Input: dimensioned drawing with shaded views. Units: mm. Origin: part minimum x, y, z. A direction names the side the tool comes from. Give positions to 0.01 mm unless a question says otherwise; leave off trailing zeros. Order: outer loops, then holes, each group sorted by start corner. A loop starts at its lowest first (then second) coordinate and runs counter-clockwise, first axis right, second up. Notation, with made-up numbers: (52, -1) -> (104, -1) arc R30 cw to (104, 38) -> close; hole circle Ø7 at (69, 21). An arc over 180 degrees is marked (long way). One line per question, with ' | ' between items. Start each with the question number.
(1) Set-up query: the marked faces 5 and 6. Return all of +Z, -Z, +X, -X, +Y, -Y with unobstructed straight access to the full face (end or side cutting, diameter ignored); none if empty.
(2) Mould query, pull axis X, two halves, no side actions, for the marked faces 1, 2, 3 and 4. Classes: +X half, -X half, draft (parallel to the pull), parting line (faces both ways), or undercut.
(3) Section B-B (x = 4.75). Return loops of the section in (y, z), then the cut area to 3 significant figures.
(4) Ray query, L1, parallel to X at y = 0.4, z = 23; L2, parallel to Y at x = 10, z = 41; L3, parallel to Z at x = 12.75, y = 2.9. Return the intervals inside material, ascending.
(5) First-contact query: pin 1 Ø2 at (x, y) = (9, 1.5) entering from -Z; pin 2 Ø3 at (x, z) = (10.5, 23.5) entering from -Y; pin 3 Ø3.5 at (x, y) = (12, 2) entering from +Z. Flat tips, straight axial feed; report the tip coordinate or a pass-through.
(6) Section C-C (y = 2.45). Return loops of the section in (x, z).
(7) Section A-A (z = 40). Return loops of the section in (x, y), then the cut area to 3 significant figures.
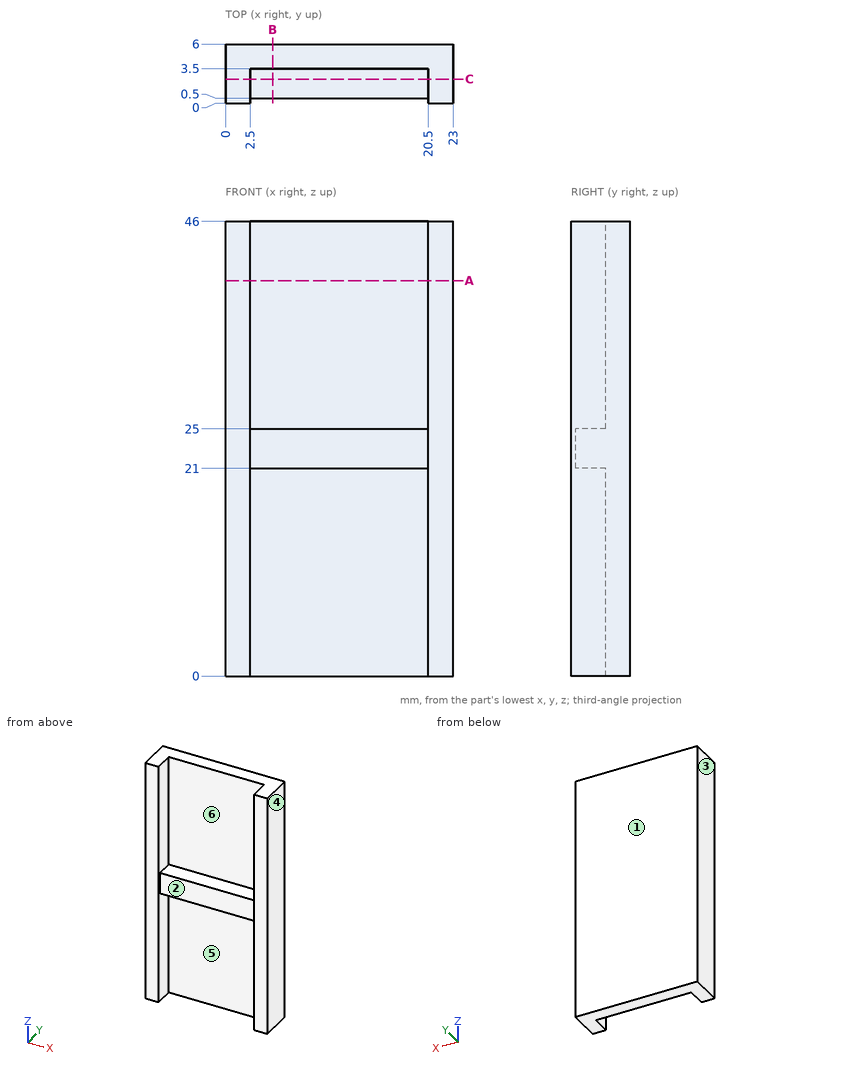
Response:
1) face 5: -Z, -Y | face 6: +Z, -Y
2) face 1: draft | face 2: undercut | face 3: -X half | face 4: +X half
3) outline: (0.5, 21) -> (3.5, 21) -> (3.5, 0) -> (6, 0) -> (6, 46) -> (3.5, 46) -> (3.5, 25) -> (0.5, 25) -> close | area: 127 mm^2
4) L1: x = 0 to 2.5, 20.5 to 23 | L2: y = 3.5 to 6 | L3: z = 21 to 25
5) pin 1: stops at z = 21 | pin 2: stops at y = 0.5 | pin 3: stops at z = 46
6) outline: (0, 0) -> (2.5, 0) -> (2.5, 21) -> (20.5, 21) -> (20.5, 0) -> (23, 0) -> (23, 46) -> (20.5, 46) -> (20.5, 25) -> (2.5, 25) -> (2.5, 46) -> (0, 46) -> close
7) outline: (0, 0) -> (2.5, 0) -> (2.5, 3.5) -> (20.5, 3.5) -> (20.5, 0) -> (23, 0) -> (23, 6) -> (0, 6) -> close | area: 75.0 mm^2
